```python
from build123d import *

# Parameters (mm, degrees)
F2_SIZE  = 5
F3_SIZE2 = 2
F3_SIZE  = 4
F4_R     = 1
F5_R     = 1.575
F6_DEPTH = 1.8
F7_R     = 5


with BuildPart() as f1:
    # F0 (on Front) → F1 (revolve)
    with BuildSketch(Plane.XZ):
        Polygon((0, 41), (0, 0), (2.2364340257, 0), (2.2364340257, 1.25), (13.85, 1.25), (13.85, 27.25), (4.4, 27.25), (4.4, 31), (1.5875, 31), (1.5875, 41), align=None)
    revolve(axis=Axis((0, 0, 53.8787767291), (0, 0, 1)))

    # F2
    f2_edges = [f1.edges().sort_by_distance(p)[0] for p in [
        (-13.85, 0, 27.25),
    ]]
    chamfer(f2_edges, length=F2_SIZE)

    # F3
    f3_edges = [f1.edges().sort_by_distance(p)[0] for p in [
        (-13.85, 0, 1.25),
    ]]
    f3_side = f1.faces().sort_by_distance((-13.85, 0, 11.75))[0]
    chamfer(f3_edges, length=F3_SIZE, length2=F3_SIZE2, reference=f3_side)

    # F4
    f4_edges = [f1.edges().sort_by_distance(p)[0] for p in [
        (-4.4, 0, 31),
    ]]
    fillet(f4_edges, radius=F4_R)

    # F5 (on face) → F6 (join)
    with BuildSketch(Plane(origin=(0, 0, 1.25), x_dir=(1, 0, 0), z_dir=(0, 0, -1))):
        with BuildLine():
            Line((-3.5, 3.5), (-17.075, 3.5))
            ThreePointArc((-17.075, 3.5), (-20.575, 0), (-17.075, -3.5))
            Line((-17.075, -3.5), (-3.5, -3.5))
            Line((-3.5, -3.5), (-3.5, -17.075))
            ThreePointArc((-3.5, -17.075), (0, -20.575), (3.5, -17.075))
            Line((3.5, -17.075), (3.5, -3.5))
            Line((3.5, -3.5), (17.075, -3.5))
            ThreePointArc((17.075, -3.5), (20.575, 0), (17.075, 3.5))
            Line((17.075, 3.5), (3.5, 3.5))
            Line((3.5, 3.5), (3.5, 17.075))
            ThreePointArc((3.5, 17.075), (0, 20.575), (-3.5, 17.075))
            Line((-3.5, 17.075), (-3.5, 3.5))
        make_face()
        with Locations((0, -17.075)):
            Circle(F5_R, mode=Mode.SUBTRACT)
        with Locations((-17.075, 0)):
            Circle(F5_R, mode=Mode.SUBTRACT)
        with Locations((17.075, 0)):
            Circle(F5_R, mode=Mode.SUBTRACT)
        with Locations((0, 17.075)):
            Circle(F5_R, mode=Mode.SUBTRACT)
    extrude(amount=F6_DEPTH)

    # F7
    f7_edges = [f1.edges().sort_by_distance(p)[0] for p in [
        (-3.5, -3.5, 0.35),
        (-3.5, 3.5, 0.35),
        (3.5, 3.5, 0.35),
        (3.5, -3.5, 0.35),
    ]]
    fillet(f7_edges, radius=F7_R)


solid = f1.part
```
Geometry check sheet. Reference: the model listing, model coordinates, mm. A direction names the side the tool comes from. Coordinates: 2 decimals unless noted, no trailing zeros. Loops run counter-clockwise (first coordinate to the right, second up) from the corner with the lowest first, then second, coordinate; pieces in that order, holes last. Notation, with made-up numbers: (-6, 37.25) - (29, 37.25) arc R28 ccw to (29, 67.25) - close; hole circle Ø4 at (-5.5, 3). An arc over 180 degrees is marked (long way). One line per item, written item: value. Start each with the question number.
(1) Depth check by flat-ended pin: P1, Ø0.9, axis at y = -13.5, z = 0.5, coming from the -X side; P2, Ø3.5, axis at x = -17.075, y = 0, coming from the -Z side; P3, Ø2, axis at x = -12, z = 26.5, coming from the +Y side; P4, Ø0.9, axis at x = 14.5, z = 0, coming from the -Y side. Enter the tip coordinate at first touch or a pass-through.
(2) Cross-section at C-C on z = 33. Enter the section's corners in (x, y) (1 decimal), plus the area to 3 significant figures.
(3) Tool access check on faces 5 (the flat face through (-3.5, -13, 0)), 6 (the flat face through (13, -3.5, 0)), 7 (the flat face through (7, 7, 1.25)), 8 (the flat face through (-2.1, 4.1, 27.25)). Record the directions out of +Z, -Z, +X, -X, +Y, -Y that give a thin tool (end or side, any length) a straight path to the whole face; none if there is none.
(4) Material ranges on line 1 (X direction, y = 0, z = 0.65) (3 decimals); line 2 (Z direction, x = -2, y = 2), recorded low to high. Write a range as [from, to].
(5) Mould release check, pull along Z, two halves, no side actions. Record for faces 1 (the flat face through (-6, 7, 1.25)), 2 (the conical face through (-9.48, -7.27, 1.44)), 3 (the flat face through (-3.5, 13, 0)), 4 (the flat face through (-2, -1, 31)): released by +Z, released by -Z, zero draft, split by the parting line, or undercut.
(6) Cross-section at A-A on x = 0. Count the separate pieces of the cut face and the enclosed holes in it, plus the area to 3 significant figures.
Results below:
1. P1: stops at x = -3.5
1. P2: stops at z = -0.55
1. P3: passes through
1. P4: stops at y = -3.5
2. outline: circle Ø3.2 at (0, 0)
2. area: 7.92 mm2
3. face 5: -Z, -X, -Y
3. face 6: -Z, +X, -Y
3. face 7: -Z, +X, +Y
3. face 8: +Z
4. line 1: x = [-20.575, -18.65], [-15.5, 15.5], [18.65, 20.575]
4. line 2: z = [-0.55, 31]
5. face 1: released by -Z
5. face 2: undercut
5. face 3: zero draft
5. face 4: released by +Z
6. separate pieces: 3
6. enclosed holes: 0
6. area: 814 mm2
